Part model, mm, in its own coordinate system. A direction names the side the tool comes from. Round coordinates to 2 decimals unless told otherwise and drop trailing zeros. Write each loop counter-clockwise with the first axis right and the second up, starting at its lowest first coordinate (ties: lowest second). Pieces come first, ordered by that corner, then holes.
1) Flat gauge pins, fed straight in: pin 1 (4 mm diameter, centred on y = 31.75, z = 44.45, fed in from +X); pin 2 (1.4 mm diameter, centred on x = 1, z = 30.5, fed in from +Y); pin 3 (3 mm diameter, centred on x = 0, z = 6.35, fed in from -Y); pin 4 (5 mm diameter, centred on x = -1, z = 43.5, fed in from -Y). Where does each tip first touch, or does it go through?
2) Which spindle directions (+Z, -Z, +X, -X, +Y, -Y) get a long thin tool onto all of the face, cutting with end or side? Do faces 5 (the cylindrical face through (-0.11, -31.66, 59.75)), 6 (the flat face through (0, 29, 31)), 7 (the flat face through (-6.35, 1, 31)). Say none if no direction does.
3) Saw through at B-B on x = -1. Count the separate pieces of the cut face and the enclosed holes in it, and give its area (3 significant figures).
4) Drill centre lines: L1, parallel to X at y = 26, z = 44.5; L2, parallel to X at y = -29.75, z = 57.15; L3, parallel to Y at x = -0.5, z = 30.5. Where is each one in solid material? Low to high.
5) Saw through at A-A on z = 31.75. Write the cut outline in (x, y), and give its area (3 significant figures).
6) Pull direction Z, two halves, no side cores. Call faces 1 (the flat face through (0, 1, 63.5)), 2 (the flat face through (0, -38.1, 31)), 3 (the flat face through (0, 1, 0)), 4 (the conical face through (0.136, -24.107, 5.919)): +Z half, -Z half, draft (parallel to the pull), parting line (faces both ways), or undercut.
Autodesk Inventor part; units mm, degrees
ref_plane "YZ Plane" through (0, 0, 0) normal (1, 0, 0) x (0, 1, 0)
ref_plane "XZ Plane" through (0, 0, 0) normal (0, 1, 0) x (-1, 0, 0)
ref_plane "XY Plane" through (0, 0, 0) normal (0, 0, 1) x (1, 0, 0)
sketch "Sketch1" plane through (0, 0, 0) normal (0, 0, 1) x (1, 0, 0)
  line L0 (-6.35, -38.1) -> (6.35, -38.1)
  line L1 (6.35, -38.1) -> (6.35, 38.1)
  line L2 (6.35, 38.1) -> (-6.35, 38.1)
  line L3 (-6.35, 38.1) -> (-6.35, -38.1)
  line L4 (-6.35, -38.1) -> (6.35, 38.1) construction
  line L5 (6.35, -38.1) -> (-6.35, 38.1) construction
  line L6 (-0.889, 50.8) -> (0.889, 50.8)
  line L7 (0.889, 50.8) -> (0.889, 25.4)
  line L8 (0.889, 25.4) -> (-0.889, 25.4)
  line L9 (-0.889, 25.4) -> (-0.889, 50.8)
  line L10 (-0.889, 50.8) -> (0.889, 25.4) construction
  line L11 (0.889, 50.8) -> (-0.889, 25.4) construction
  point P0 (0, 0)
  point P1 (0, 38.1)
  dimension "d0" = 12.7
  dimension "d1" = 76.2
  dimension "d2" = 1.778
  dimension "d3" = 12.7
extrude "Extrusion1" add sketch "Sketch1" along normal blind 63.5 contours L3 L2 L9 L8 L7 L1 L0 | L2 L7 L8 L9
sketch "Sketch2" plane through (0, 0, 0) normal (0, 0, -1) x (-1, 0, 0)
  line L0 (-6.35, 38.1) -> (6.35, 38.1)
  line L1 (0, 38.1) -> (-1.778, 38.1)
  line L2 (-1.778, 38.1) -> (-1.778, 25.4)
  line L3 (-1.778, 25.4) -> (0, 25.4)
  line L4 (0, 25.4) -> (0, 38.1)
  point P0 (0, 0)
  dimension "d6" = 1.778
  dimension "d7" = 12.7
extrude "Extrusion2" cut sketch "Sketch2" against normal blind 63.5
sketch "Sketch3" plane through (6.35, -38.1, 0) normal (1, 0, 0) x (0, 0, -1)
  line L0 (0, 76.2) -> (-63.5, 76.2)
  line L1 (-63.5, 0) -> (-63.5, 76.2)
  point P0 (0, 38.1)
  point P1 (-31.75, 69.85)
  dimension "d10" = 6.35
  dimension "d11" = 31.75
hole "Hole1" at (6.35, 31.75, 31.75) direction (-1, 0, 0) diameter 3.175 end through all
sketch "Sketch4" plane through (6.35, -38.1, 0) normal (1, 0, 0) x (0, 0, -1)
  line L0 (-44.45, 69.8514) -> (-19.05, 69.8514)
  line L1 (0, 0) -> (0, 76.2)
  point P0 (0, 38.1)
  dimension "d19" = 25.4
  dimension "d20" = 19.05
hole "Hole2" at (6.35, 31.7514, 44.45) at (6.35, 31.7514, 19.05) direction (-1, 0, 0) diameter 4.9784 depth 19.05 tip angle 118
sketch "Sketch5" plane through (-6.35, -38.1, 0) normal (0, -1, 0) x (1, 0, 0)
  line L0 (6.35, 63.5) -> (6.35, 0)
  line L1 (6.35, 57.15) -> (6.35, 6.35)
  dimension "d28" = 50.8
  dimension "d29" = 6.35
hole "Hole3" at (0, -38.1, 57.15) at (0, -38.1, 6.35) direction (0, 1, 0) diameter 5.207 depth 12.7 tip angle 118
sketch "Sketch6" plane through (-6.35, -38.1, 0) normal (0, -1, 0) x (1, 0, 0)
  point P0 (6.35, 0)
sketch "Sketch7" plane through (-6.35, -38.1, 0) normal (0, -1, 0) x (1, 0, 0)
  line L0 (6.35, 63.5) -> (6.35, 0)
  line L1 (6.35, 44.45) -> (6.35, 19.05)
  line L2 (0, 63.5) -> (12.7, 63.5)
  dimension "d37" = 25.4
  dimension "d38" = 19.05
hole "Hole4" at (0, -38.1, 44.45) at (0, -38.1, 19.05) direction (0, 1, 0) diameter 9.525 depth 5.334 tip angle 118
properties part number "mask holder"
Completed:
1. pin 1: passes through
1. pin 2: stops at y = 25.4
1. pin 3: stops at y = -24.74
1. pin 4: stops at y = -32.24
2. face 5: -Y
2. face 6: +Z, -Z, +Y
2. face 7: +Z, -Z, -X, +Y, -Y
3. separate pieces: 1
3. enclosed holes: 3
3. area: 4,540 mm2
4. L1: x = -6.35 to 0, 1.78 to 6.35
4. L2: x = -6.35 to -2.6, 2.6 to 6.35
4. L3: y = -38.1 to 30.77, 32.73 to 38.1
5. outline: (-6.35, -38.1) - (6.35, -38.1) - (6.35, 30.16) - (1.78, 30.16) - (1.78, 25.4) - (0, 25.4) - (0, 30.16) - (-6.35, 30.16) - close; (-6.35, 33.34) - (0, 33.34) - (0, 38.1) - (-6.35, 38.1) - close; (1.78, 33.34) - (6.35, 33.34) - (6.35, 38.1) - (1.78, 38.1) - close
5. area: 910 mm2
6. face 1: +Z half
6. face 2: draft
6. face 3: -Z half
6. face 4: undercut
